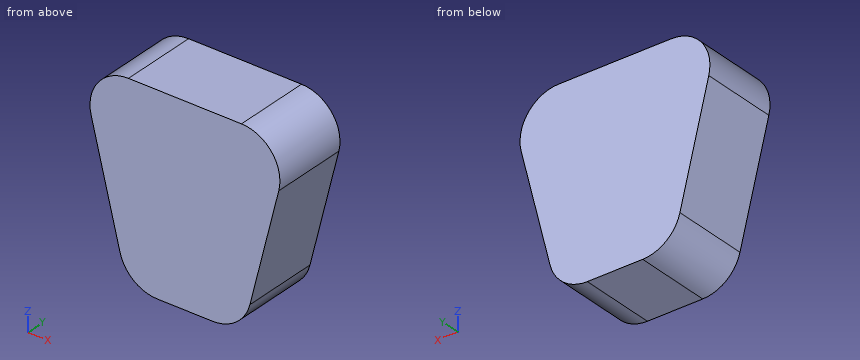
from build123d import *

# Parameters (mm, degrees)
FSHAPE1_DEPTH = 20
FRSHAPE1_R    = 10


with BuildPart() as part:
    # SShape1 → FShape1 (new body)
    with BuildSketch(Plane(origin=(0, 0, 0), x_dir=(1, 0, 0), z_dir=(0, 1, 0))):
        Polygon((-15, 25), (15, 25), (27.5, -25), (-27.5, -25), align=None)
    extrude(amount=FSHAPE1_DEPTH)

    # FRShape1
    frshape1_edges = [part.edges().sort_by_distance(p)[0] for p in [
        (-15, 10, -25),
        (15, 10, -25),
        (27.5, 10, 25),
        (-27.5, 10, 25),
    ]]
    fillet(frshape1_edges, radius=FRSHAPE1_R)


solid = part.part
Input: part model. Units: mm. Frame: model coordinates. Coordinates: 2 decimals unless noted, no trailing zeros. Loops run counter-clockwise (first coordinate to the right, second up) from the corner with the lowest first, then second, coordinate; pieces in that order, holes last.
Q1. Contact query for flat-ended pins moving along their axis: pin 1 (1 mm diameter, centred on y = 9.5, z = -16, fed in from +X) (3 decimals); pin 2 (8 mm diameter, centred on x = 15, y = 12.5, fed in from -Z); pin 3 (6 mm diameter, centred on y = 9, z = 2.5, fed in from -X) (3 decimals). Output: stop coordinate, or through.
Q2. Cut plane B-B (z = 0). Output: boundary loops of the cut face in (x, y).
Q3. Material intervals for line 1 (Z direction, x = -7.5, y = 15); line 2 (Z direction, x = -14, y = 4.5); line 3 (X direction, y = 1.25, z = 3.5) (3 decimals), sorted ascending.
Q4. Cut plane C-C (x = -17.5). Output: boundary loops of the cut face in (y, z), then the cut area to 3 significant figures.
Q5. Cut plane A-A (y = 2.5). Output: boundary loops of the cut face in (x, z).
Working result:
1. pin 1: stops at x = 17.375
1. pin 2: stops at z = -24.25
1. pin 3: stops at x = -22.625
2. outline: (-21.25, 0) - (21.25, 0) - (21.25, 20) - (-21.25, 20) - close
3. line 1: z = -25 to 25
3. line 2: z = -22.32 to 25
3. line 3: x = -22.125 to 22.125
4. outline: (0, -15) - (20, -15) - (20, 24.6) - (0, 24.6) - close
4. area: 792 mm2
5. outline: (-24.39, 12.57) - (-16.89, -17.43) arc R10 ccw to (-7.19, -25) - (7.19, -25) arc R10 ccw to (16.89, -17.43) - (24.39, 12.57) arc R10 ccw to (14.69, 25) - (-14.69, 25) arc R10 ccw to start
